from build123d import *

# Parameters (mm, degrees)
BOSS_EXTRU_2_DEPTH      = 9
ENL_V_MAT_EXTRU_2_DEPTH = 9
ENL_V_MAT_EXTRU_3_DEPTH = 10


with BuildPart() as part:
    # Esquisse2 → Boss.-Extru.2 (new body)
    with BuildSketch(Plane.XY):
        with BuildLine():
            Line((0, 0), (-1055.446290734, 0))
            add(Edge.make_bspline(
                [(-1055.446290734, 0), (-1207.572733387, 59.072106031), (-1304.579199027, 189.593529265)],
                knots=[0, 0, 0, 1, 1, 1], degree=2))
            Line((-1304.579199027, 189.593529265), (-1328.155601237, 242.090877604))
            Line((-1328.155601237, 242.090877604), (-1348.517039509, 262.446992266))
            Line((-1348.517039509, 262.446992266), (-1348.517039509, 299.331021292))
            Line((-1348.517039509, 299.331021292), (-1337.24264668, 310.608362644))
            Line((-1337.24264668, 310.608362644), (-1275.966827179, 302.644588826))
            add(Edge.make_bspline(
                [(-1275.966827179, 302.644588826), (-1212.760641583, 141.531535954), (-1050.525159664, 78.394553502)],
                knots=[0, 0, 0, 1, 1, 1], degree=2))
            Line((-1050.525159664, 78.394553502), (-46.371074076, 78.394553502))
            Line((-46.371074076, 78.394553502), (48.76008987, 228.44376205))
            Line((48.76008987, 228.44376205), (115.880348206, 284.547364773))
            Line((115.880348206, 284.547364773), (175.286334456, 328.432610938))
            Line((175.286334456, 328.432610938), (175.286334456, 257.621549377))
            Line((175.286334456, 257.621549377), (107.11594567, 180.577636332))
            Line((107.11594567, 180.577636332), (0, 0))
        make_face()
    extrude(amount=BOSS_EXTRU_2_DEPTH)

    # Esquisse4 → Enlèv. mat.-Extru.2 (cut)
    with BuildSketch(Plane.XY.offset(9)):
        Polygon((-1192.710056644, 217.724215408), (-1192.710056644, 117.812636738), (-1186.710056644, 117.812636738), (-1186.710056644, 209.090265158), (-1144.70133954, 205.492785887), (-1111.824911273, 179.590935136), (-1111.824911273, 55.314515649), (-1105.824911273, 55.314515649), (-1105.824911273, 174.913937406), (-1058.771084869, 188.659470271), (-1027.191161845, 161.497477767), (-1027.191161845, 30), (-1021.191161845, 30), (-1021.191161845, 167.225098507), (-976.159938867, 174.429619005), (-943.229008237, 161.127659365), (-943.229008237, 30), (-937.229008237, 30), (-937.229008237, 164.093815562), (-899.191490776, 172.001101596), (-861.857811784, 160.098627493), (-861.857811784, 30), (-855.857811784, 30), (-855.857811784, 196.236545153), (-815.986169177, 204.901610664), (-775.188433973, 184.176190605), (-775.188433973, 30), (-769.188433973, 30), (-769.188433973, 176.450577912), (-732.223715867, 183.004336583), (-693.639593808, 163.215620457), (-693.639593808, 30), (-687.639593808, 30), (-687.639593808, 172.485228345), (-653.152535866, 182.871939208), (-610.716601792, 161.453305285), (-610.716601792, 30), (-604.716601792, 30), (-604.716601792, 256.125318922), (-551.321272632, 268.910222611), (-528.666744333, 255.862211449), (-528.666744333, 34.3), (-522.666744333, 34.3), (-522.666744333, 255.102102604), (-476.392141731, 269.107524931), (-444.607914754, 258.656296952), (-444.607914754, 36.7), (-438.607914754, 36.7), (-438.607914754, 253.443093933), (-391.056155042, 266.894918017), (-360.02126631, 254.206439852), (-360.02126631, 30), (-354.02126631, 30), (-354.02126631, 250.104032237), (-303.804875297, 262.547483763), (-275.81856885, 247.243298089), (-275.81856885, 39.1), (-269.81856885, 39.1), (-269.81856885, 230.071554094), (-217.437093626, 257.378680484), (-192.806508582, 246.762372601), (-192.806508582, 38.7), (-186.806508582, 38.7), (-186.806508582, 245.622867868), (-134.999273909, 264.79720393), (-106.993498927, 255.334085011), (-106.993498927, 46.1), (-100.993498927, 46.1), (-100.993498927, 258.655280604), (-22.735685337, 264.839286488), (-22.735685337, 88.7), (-16.735685337, 88.7), (-16.735685337, 231.395876397), (-1.733463181, 266.202092714), (54.176868866, 313.052154508), (54.176868866, 197.147050424), (60.176868866, 197.147050424), (60.176868866, 330.337520125), (-1075.947973634, 334.662873451), align=None)
    extrude(amount=-ENL_V_MAT_EXTRU_2_DEPTH, mode=Mode.SUBTRACT)

    # Esquisse5 → Enlèv. mat.-Extru.3 (cut)
    with BuildSketch(Plane.XY.offset(9)):
        Polygon((169.286334456, 324.000204482), (169.286334456, 281.800204482), (175.286334456, 281.800204482), (202.680394495, 285.052171219), (208.588297758, 339.079823363), (181.275473189, 338.718158681), align=None)
    extrude(amount=-ENL_V_MAT_EXTRU_3_DEPTH, mode=Mode.SUBTRACT)


solid = part.part
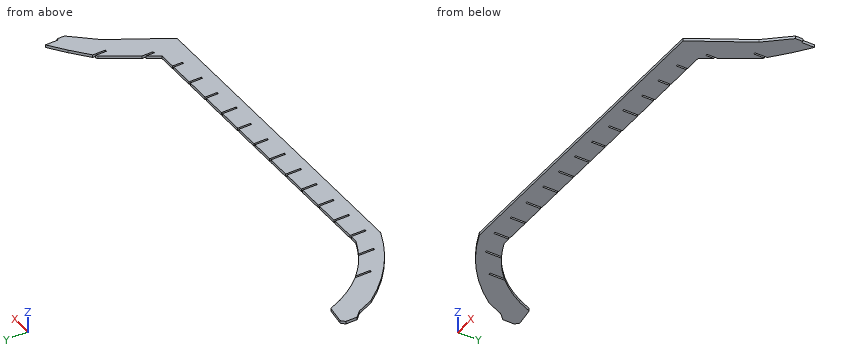
Work out the finished part from the listing and answer in its coordinate system (mm). Give positions to 0.01 mm unless a question says otherwise; leave off trailing zeros. Order: outer loops, then holes, each group sorted by start corner. A loop starts at its lowest first (then second) coordinate and runs counter-clockwise, first axis right, second up. Notation, with made-up numbers: (0.5, 31.25) - (42.5, 31.25) arc R23 cw to (42.5, 61.25) - close; hole circle Ø7 at (-2.75, 4.25). An arc over 180 degrees is marked (long way). Answer as CSV lines item,"result". Start each with the question number.
Q1. The part is cut by section B-B (y = 214). Give the number of separate pieces and of enclosed holes in the cut face, then the cut area to 3 significant figures.
Q2. The part is cut by section A-A (x = -72). Write down the section's boundary in (y, z), then the cut area to 3 significant figures.
Q3. Find the intervals of material crossed by L1, parallel to X at y = 162, z = 8.5; L2, parallel to X at y = 163.5, z = 4.75; L3, parallel to Y at x = -992.5, z = 5.5, in increasing order. Write a range as [from, to].
Q4. Given pin 1 Ø4 at (x, z) = (12.5, 4.5) entering from +Y; pin 2 Ø10 at (x, y) = (-48, 60.5) entering from -Z; pin 3 Ø3 at (x, z) = (172.5, 6) entering from +Y; pin 4 Ø4 at (x, z) = (-693, 2) entering from +Y, each flat-ended and moving along its own axis, determine where each tip first touches the part or whether it passes through.
Check result:
1,separate pieces,"3"
1,enclosed holes,"0"
1,area,"1,600 mm²"
2,outline,"(0, 0) - (78.39, 0) - (78.39, 9) - (0, 9) - close"
2,area,"706 mm²"
3,L1,"x = [-1282.79, -1192.71], [-1186.71, -1183.89], [6.63, 96.1]"
3,L2,"x = [-1284.04, -1192.71], [-1186.71, -1185.44], [7.59, 96.99]"
3,L3,"y = [0, 78.39]"
4,pin 1,"stops at y = 174.41"
4,pin 2,"stops at z = 0"
4,pin 3,"stops at y = 281.8"
4,pin 4,"stops at y = 78.39"
